from build123d import *

# Parameters (mm, degrees)
F0_W      = 990.5
F0_H      = 12
F1_DEPTH  = 899
F2_W      = 9.5
F2_H      = 6
F3_DEPTH  = 899.001
F4_W      = 6
F4_H      = 6
F5_DEPTH  = 899.001
F6_W      = 6
F6_H      = 12.5
F7_DEPTH  = 990.501
F9_DEPTH  = 990.501
F11_DEPTH = 12.001


with BuildPart() as f1:
    # F0 (on Top) → F1 (new body)
    with BuildSketch(Plane.XY):
        with Locations((495.25, -6)):
            Rectangle(F0_W, F0_H)
    extrude(amount=F1_DEPTH)

    # F2 (on Top) → F3 (cut, through all)
    with BuildSketch(Plane.XY):
        with Locations((4.75, -9)):
            Rectangle(F2_W, F2_H)
    extrude(amount=F3_DEPTH, mode=Mode.SUBTRACT)

    # F4 (on Top) → F5 (cut, through all)
    with BuildSketch(Plane.XY):
        with Locations((981.5, -9)):
            Rectangle(F4_W, F4_H)
    extrude(amount=F5_DEPTH, mode=Mode.SUBTRACT)

    # F6 (on Right) → F7 (cut, through all)
    with BuildSketch(Plane.YZ):
        with Locations((-9, 116.25)):
            Rectangle(F6_W, F6_H)
    extrude(amount=F7_DEPTH, mode=Mode.SUBTRACT)

    # F8 (on Right) → F9 (cut, through all)
    with BuildSketch(Plane.YZ):
        Polygon((-25, 0), (0, 0), (0, 109), (-6.915434, 90), (-25, 90), align=None)
    extrude(amount=F9_DEPTH, mode=Mode.SUBTRACT)

    # F10 (on face) → F11 (cut, through all)
    with BuildSketch(Plane.XZ.offset(12)):
        Polygon((983.584566, 90), (990.5, 90), (990.5, 109), align=None)
    extrude(amount=-F11_DEPTH, mode=Mode.SUBTRACT)


solid = f1.part
The model under review builds one solid part; all positions refer to its coordinate system, in mm. Round coordinates to 2 decimals unless told otherwise and drop trailing zeros. Loops run counter-clockwise (first coordinate to the right, second up) from the corner with the lowest first, then second, coordinate; pieces in that order, holes last. Notation, with made-up numbers: M 41.25,-6.5 L 80.25,-6.5 A20 cw 80.25,2.5 Z; hole C -3,-39.5 d7. An arc over 180 degrees is marked long. Answer as CSV lines item,"result". Start each with the question number.
Item 1: Consider section A-A (y = -9.5). Write out the cut boundary in (x, z), then the cut area to 3 significant figures.
Item 2: Insertion check: P1, Ø6.5, axis at y = -9.5, z = 104, coming from the -X side; P2, Ø1.8, axis at y = -9.5, z = 100.5, coming from the +X side; P3, Ø1.5, axis at x = 104, z = 250.5, coming from the +Y side. Each pin has a flat end and moves straight along its axis. Give the tip position at first contact, or say it passes through.
Item 3: Wall thickness on line 1 (Z direction, x = 817, y = -11.25); line 2 (X direction, y = -9.75, z = 853): over which ranges is each line inside the solid? List them lowest first. Write a range as [from, to].
Answer:
1,outline,"M 9.5,90 L 978.5,90 L 978.5,110 L 9.5,110 Z; M 9.5,122.5 L 978.5,122.5 L 978.5,899 L 9.5,899 Z; M 984.5,92.52 L 990.5,109 L 990.5,110 L 984.5,110 Z; M 984.5,122.5 L 990.5,122.5 L 990.5,899 L 984.5,899 Z"
1,area,"777,000 mm^2"
2,P1,"stops at x = 9.5"
2,P2,"stops at x = 987.73"
2,P3,"stops at y = 0"
3,line 1,"z = [90, 110], [122.5, 899]"
3,line 2,"x = [9.5, 978.5], [984.5, 990.5]"
